Read the model definition and answer for the solid it produces. Units are mm, in the model's axes. Face numbers are marked on the shaded views. A direction names the side the tool comes from. Give positions to 0.01 mm unless a question says otherwise; leave off trailing zeros. Order: outer loops, then holes, each group sorted by start corner. A loop starts at its lowest first (then second) coordinate and runs counter-clockwise, first axis right, second up. Notation, with made-up numbers: (23, -13) - (45, -13) arc R12 ccw to (45, -4) - close; hole circle Ø3 at (-20, 28). An arc over 180 degrees is marked (long way). Write item = value, one per line.
```python
from build123d import *

# Parameters (mm, degrees)
SKETCH_1_W      = 4
SKETCH_1_H      = 5.856888772
SKETCH_1_R      = 0.999999985
EXTRUDE_1_DEPTH = 3
SKETCH_2_R      = 1.5
EXTRUDE_2_DEPTH = 1.5


with BuildPart() as part:
    # 草图1 → 凸台-拉伸1 (new body)
    with BuildSketch(Plane.XY):
        Rectangle(SKETCH_1_W, SKETCH_1_H)
        Circle(SKETCH_1_R, mode=Mode.SUBTRACT)
    extrude(amount=EXTRUDE_1_DEPTH)

    # 草图2 → 凸台-拉伸2 (add)
    with BuildSketch(Plane(origin=(0, 2.928444386, 0), x_dir=(1, 0, 0), z_dir=(0, 1, 0))):
        with Locations(Location((0, -1.5, 0), (0, 0, 270))):
            Circle(SKETCH_2_R)
    extrude_2 = extrude(amount=EXTRUDE_2_DEPTH)

    # 镜向1: 凸台-拉伸2 across plane
    add(extrude_2.mirror(Plane.ZX))


solid = part.part
```
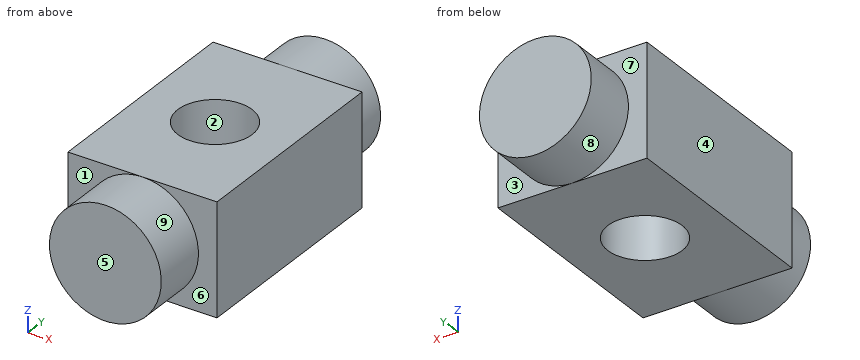
1. A flat-ended cylindrical pin translates along its axis: pin 1 (0.6 mm diameter, centred on x = 1.5, z = 2, fed in from +Y). Find the tip coordinate at first contact, or state that the pin passes through.
Recorded:
pin_1 = 4.43
2. Section C-C (x = 1.75) is taken. Determine the outline of the cut face in (y, z), and give its area (3 significant figures).
Recorded:
outline = (-2.93, 0) - (2.93, 0) - (2.93, 3) - (-2.93, 3) - close
area = 17.6 mm^2
3. Section A-A (y = 0) is taken. Determine the outline of the cut face in (x, z).
Recorded:
outline = (-2, 0) - (-1, 0) - (-1, 3) - (-2, 3) - close; (1, 0) - (2, 0) - (2, 3) - (1, 3) - close
4. Determine the mould class of the marked faces 1, 2, 3 and 4 for opening direction Y: +Y half, -Y half, draft (parallel to the pull), parting line (faces both ways), or undercut.
Recorded:
face_1 = -Y half
face_2 = undercut
face_3 = +Y half
face_4 = draft
5. Section D-D (y = -3.5) is taken. Determine the outline of the cut face in (x, z).
Recorded:
outline = circle Ø3 at (0, 1.5)
6. For the marked faces 5, 6, 7, 8 and 9, determine the directions among +Z, -Z, +X, -X, +Y, -Y from which every point of the face is accessible in a straight line to the end or side of a thin tool.
Recorded:
face_5 = +Z, -Z, +X, -X, -Y
face_6 = +X, -Y
face_7 = -X, +Y
face_8 = +Y
face_9 = -Y
7. Straight lines are drawn through the part: L1, parallel to Y at x = 0, z = 2.1; L2, parallel to Y at x = 1.8, z = 0.2; L3, parallel to X at y = -0.5, z = 1.05. For each, find the intervals that lie inside material, in ascending order. Write a range as [from, to].
Recorded:
L1 = [-4.43, -1], [1, 4.43]
L2 = [-2.93, 2.93]
L3 = [-2, -0.87], [0.87, 2]
8. Section B-B (z = 2.85) is taken. Determine the outline of the cut face in (x, y).
Recorded:
outline = (-2, -2.93) - (-0.65, -2.93) - (-0.65, -4.43) - (0.65, -4.43) - (0.65, -2.93) - (2, -2.93) - (2, 2.93) - (0.65, 2.93) - (0.65, 4.43) - (-0.65, 4.43) - (-0.65, 2.93) - (-2, 2.93) - close; hole circle Ø2 at (0, 0)
